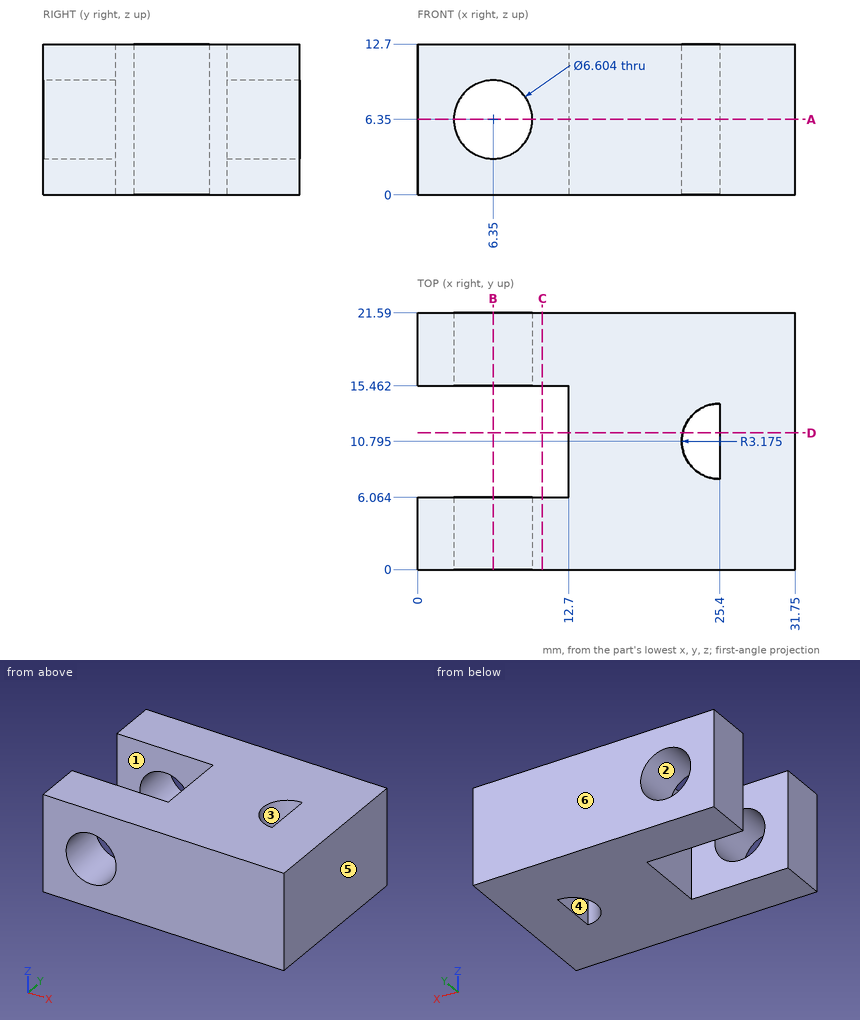
Answer from the drawing. Dimensions are ordinates in mm from the lowest x, y and z of the part. A direction names the side the tool comes from. Give positions to 0.01 mm unless a question says otherwise; leave off trailing zeros. Order: outer loops, then holes, each group sorted by start corner. A loop starts at its lowest first (then second) coordinate and runs counter-clockwise, first axis right, second up. Notation, with made-up numbers: (81.5, 89) -> (124.5, 89) arc R15 ccw to (124.5, 109) -> close; hole circle Ø4 at (47.25, 48). An arc over 180 degrees is marked (long way). Answer as a JSON object with one key per item and string values. Group by question number.
1. Section B-B on x = 6.35 is taken. Determine the outline of the cut face in (y, z), plus the area to 3 significant figures.
2. Section D-D on y = 11.5 is taken. Determine the outline of the cut face in (x, z).
3. Section C-C on x = 10.5 is taken. Determine the outline of the cut face in (y, z), plus the area to 3 significant figures.
4. A flat-ended cylindrical pin translates along its axis: pin 1 Ø3 at (y, z) = (11, 4) entering from -X. Find the tip coordinate at first contact, or state that the pin passes through.
5. Consider line 1 along Y through (x, z) = (7.5, 1); line 2 along X through (y, z) = (4.75, 6.35); line 3 along X through (y, z) = (12.5, 6.5). Determine where each line is inside the solid, lowest interval first. Write a range as [from, to].
6. A tool of negligible diameter and unlimited length cuts with its end or side. For the marked faces 1, 2 and 3, from which of +Z, -Z, +X, -X, +Y, -Y can it reach the whole face along a straight path? Write none if from no direction.
7. The mould has two halves that part along Y. Classify the marked faces 4, 5 and 6: released by +Y, released by -Y, zero draft, split by the parting line, or undercut.
8. Section A-A on z = 6.35 is taken. Determine the outline of the cut face in (x, y) (3 decimals), plus the area to 3 significant figures.
Result sheet:
{
 "1": {"outline": "(0, 0) -> (6.06, 0) -> (6.06, 3.05) -> (0, 3.05) -> close; (0, 9.65) -> (6.06, 9.65) -> (6.06, 12.7) -> (0, 12.7) -> close; (15.46, 0) -> (21.59, 0) -> (21.59, 3.05) -> (15.46, 3.05) -> close; (15.46, 9.65) -> (21.59, 9.65) -> (21.59, 12.7) -> (15.46, 12.7) -> close", "area": "74.3 mm^2"},
 "2": {"outline": "(12.7, 0) -> (22.3, 0) -> (22.3, 12.7) -> (12.7, 12.7) -> close; (25.4, 0) -> (31.75, 0) -> (31.75, 12.7) -> (25.4, 12.7) -> close"},
 "3": {"outline": "(0, 0) -> (6.06, 0) -> (6.06, 12.7) -> (0, 12.7) -> close; (15.46, 0) -> (21.59, 0) -> (21.59, 12.7) -> (15.46, 12.7) -> close", "area": "155 mm^2"},
 "4": {"pin 1": "stops at x = 12.7"},
 "5": {"line 1": "y = [0, 6.06], [15.46, 21.59]", "line 2": "x = [0, 3.05], [9.65, 31.75]", "line 3": "x = [12.7, 22.72], [25.4, 31.75]"},
 "6": {"face 1": "+Z, -Z, -X", "face 2": "+Y, -Y", "face 3": "+Z, -Z"},
 "7": {"face 4": "undercut", "face 5": "zero draft", "face 6": "released by +Y"},
 "8": {"outline": "(0, 0) -> (3.048, 0) -> (3.048, 6.064) -> (0, 6.064) -> close; (0, 15.462) -> (3.048, 15.462) -> (3.048, 21.59) -> (0, 21.59) -> close; (9.652, 0) -> (31.75, 0) -> (31.75, 21.59) -> (9.652, 21.59) -> (9.652, 15.462) -> (12.7, 15.462) -> (12.7, 6.064) -> (9.652, 6.064) -> close; hole (25.4, 7.62) -> (25.4, 13.97) arc R3.175 ccw to start", "area": "470 mm^2"}
}
